The listing builds one solid part. Answer for the finished solid, in the listing's coordinates (mm). Face numbers are marked on the shaded views. A direction names the side the tool comes from. Give positions to 0.01 mm unless a question says otherwise; leave off trailing zeros. Loops run counter-clockwise (first coordinate to the right, second up) from the corner with the lowest first, then second, coordinate; pieces in that order, holes last. Notation, with made-up numbers: (-38.75, -15.5) - (-3.75, -15.5) arc R16 cw to (-3.75, -7.5) - close; hole circle Ø8 at (-21, 64). An arc over 180 degrees is marked (long way). Write item = value, one per line. Start each with the question number.
1) Consider probe 1 along X at (y, z) = (94, 3.2); probe 2 along X at (y, z) = (94, 2.25); probe 3 along Y at (x, z) = (27.5, 1.5). Determine where each line is inside the solid, lowest interval first.
2) The part is cut by section B-B on z = 1.5. Write down the section's boundary in (x, y), plus the area to 3 significant figures.
3) Which of the six approach directions +Z, -Z, +X, -X, +Y, -Y give full straight-line access (tool end or side, diameter ignored) to the marked faces 1 and 2?
4) Flat-ended cylindrical pins translate along their axes: P1, Ø0.8, axis at y = 97, z = 3.5, coming from the +X side; P2, Ø7.5, axis at x = -94.5, y = 94.5, coming from the +Z side; P3, Ø1.3, axis at x = 27.5, y = 94, coming from the -Z side; P4, Ø3, axis at y = 100, z = 6, coming from the +X side. Find the tip coordinate at first contact, or state that the pin passes through.
5) The mould has two halves that part along X. Classify the marked faces 3 and 4: +X half, -X half, draft (parallel to the pull), parting line (faces both ways), or undercut.
6) The part is cut by section A-A on x = -105. Write down the section's boundary in (y, z).
7) The part is cut by section C-C on x = -28. Write down the section's boundary in (y, z).
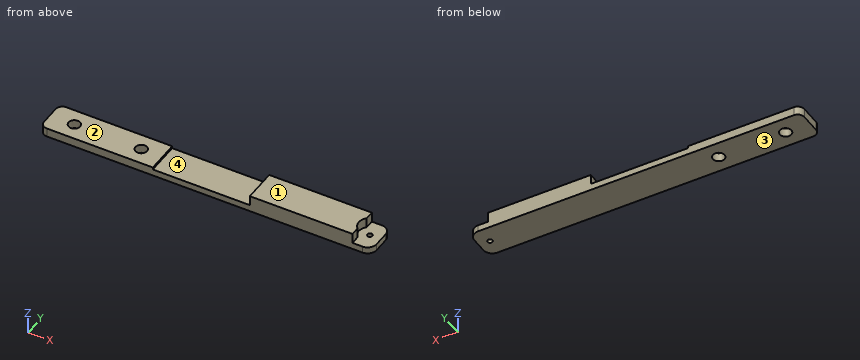
Solid Edge part; units mm, degrees
sketch "Sketch1" plane through (0, 0, 0) normal (0, 0, 1) x (1, 0, 0)
  line L0 (-116, 86.5) -> (32.5, 86.5)
  line L1 (32.5, 101.5) -> (32.5, 86.5)
  line L2 (32.5, 101.5) -> (-116, 101.5)
  line L3 (-116, 101.5) -> (-116, 86.5)
extrude "Protrusion1" add sketch "Sketch1" along normal blind 3
sketch "Sketch2" plane through (26, 94, 3) normal (0, 0, 1) x (1, 0, 0)
  circle A0 centre (1.5, 0) radius 1.1
extrude "Cutout1" cut sketch "Sketch2" against normal up to next
fillet "Round_3" radius 4 2 edges at (32.5, 86.5, 1.5) (32.5, 101.5, 1.5)
sketch "Sketch3" plane through (-41.5, 94, 3) normal (0, 0, 1) x (1, 0, 0)
  line L0 (65.5, -3.5707) -> (65.5, -7.5)
  line L1 (65.5, -7.5) -> (19.5, -7.5)
  line L2 (19.5, -7.5) -> (19.5, 7.5)
  line L3 (65.5, 7.5) -> (19.5, 7.5)
  line L4 (65.5, 7.5) -> (65.5, 3.5707)
  arc A0 (65.5, -3.5707) -> (65.5, 3.5707) centre (69, 0) cw
extrude "ExtrudedProtrusion_7" add sketch "Sketch3" along normal blind 4.5
sketch "Sketch4" plane through (-68.75, 94, 3) normal (0, 0, 1) x (1, 0, 0)
  line L0 (-47.25, 7.5) -> (3.25, 7.5)
  line L1 (3.25, 7.5) -> (3.25, -7.5)
  line L2 (-47.25, -7.5) -> (3.25, -7.5)
  line L3 (-47.25, 7.5) -> (-47.25, -7.5)
extrude "ExtrudedProtrusion_8" add sketch "Sketch4" along normal blind 1
sketch "Sketch5" plane through (-68.75, 94, 3) normal (0, 0, 1) x (1, 0, 0)
  circle A0 centre (-36.25, 0) radius 2.6
  circle A1 centre (-6.25, 0) radius 2.6
extrude "Cutout2" cut sketch "Sketch5" along normal mid plane 10.057
fillet "Round_4" radius 3 2 edges at (-116, 86.5, 2) (-116, 101.5, 2)
Answer below:
q1.probe_1 = -116 to -107.6, -102.4 to -77.6, -72.4 to -65.5, -22 to 22.5
q1.probe_2 = -116 to -107.6, -102.4 to -77.6, -72.4 to 26.4, 28.6 to 32.5
q1.probe_3 = 86.5 to 92.9, 95.1 to 101.5
q2.outline = (-116, 89.5) arc R3 ccw to (-113, 86.5) - (28.5, 86.5) arc R4 ccw to (32.5, 90.5) - (32.5, 97.5) arc R4 ccw to (28.5, 101.5) - (-113, 101.5) arc R3 ccw to (-116, 98.5) - close; hole circle Ø5.2 at (-105, 94); hole circle Ø5.2 at (-75, 94); hole circle Ø2.2 at (27.5, 94)
q2.area = 2,170 mm2
q3.face_1 = +Z, +X, -X, +Y, -Y
q3.face_2 = +Z, -X, +Y, -Y
q4.P1 = 23.83
q4.P2 = 4
q4.P3 = through
q4.P4 = 24
q5.face_3 = draft
q5.face_4 = undercut
q6.outline = (86.5, 0) - (91.4, 0) - (91.4, 4) - (86.5, 4) - close; (96.6, 0) - (101.5, 0) - (101.5, 4) - (96.6, 4) - close
q7.outline = (86.5, 0) - (101.5, 0) - (101.5, 3) - (86.5, 3) - close
